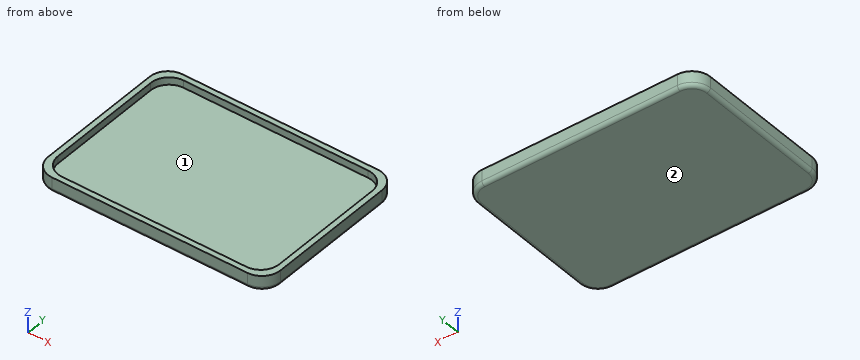
from build123d import *

# Parameters (mm, degrees)
F0_W     = 60
F0_H     = 42
F1_DEPTH = 2
F2_W     = 63
F2_H     = 45
F2_W_2   = 60
F2_H_2   = 42
F3_DEPTH = 4
F4_R     = 5
F5_R     = 1


with BuildPart() as f1:
    # F0 (on Top) → F1 (new body)
    with BuildSketch(Plane.XY):
        with Locations((30, 21)):
            Rectangle(F0_W, F0_H)
    extrude(amount=F1_DEPTH)

    # F2 (on Top) → F3 (join)
    with BuildSketch(Plane.XY):
        with Locations((30, 21)):
            Rectangle(F2_W, F2_H)
        with Locations((30, 21)):
            Rectangle(F2_W_2, F2_H_2, mode=Mode.SUBTRACT)
    extrude(amount=F3_DEPTH)

    # F4
    f4_edges = [f1.edges().sort_by_distance(p)[0] for p in [
        (-1.5, -1.5, 2),
        (61.5, -1.5, 2),
        (-1.5, 43.5, 2),
        (60, 42, 3),
        (61.5, 43.5, 2),
        (60, 0, 3),
        (0, 0, 3),
        (0, 42, 3),
    ]]
    fillet(f4_edges, radius=F4_R)

    # F5
    f5_edges = [f1.edges().sort_by_distance(p)[0] for p in [
        (30, -1.5, 0),
        (60.035534, -0.035534, 0),
        (61.5, 21, 0),
        (60.035534, 42.035534, 0),
        (30, 43.5, 0),
        (-0.035534, 42.035534, 0),
        (-1.5, 21, 0),
        (-0.035534, -0.035534, 0),
    ]]
    fillet(f5_edges, radius=F5_R)


solid = f1.part
Input: part model. Units: mm. Frame: model coordinates. Face numbers are marked on the shaded views. Round coordinates to 2 decimals unless told otherwise and drop trailing zeros. Order: outer loops, then holes, each group sorted by start corner. A loop starts at its lowest first (then second) coordinate and runs counter-clockwise, first axis right, second up.
1. Mould query, pull axis Y, two halves, no side actions, for the marked faces 1 and 2. Classes: released by +Y, released by -Y, zero draft, split by the parting line, or undercut.
The answers:
face 1: undercut
face 2: zero draft
2. Cut plane B-B, the plane x = 40. Output: boundary loops of the cut face in (y, z).
The answers:
outline: (-1.5, 1) arc R1 ccw to (-0.5, 0) - (42.5, 0) arc R1 ccw to (43.5, 1) - (43.5, 4) - (42, 4) - (42, 2) - (0, 2) - (0, 4) - (-1.5, 4) - close
3. Pin query (flat end, axial travel): P1, Ø10, axis at x = 47.5, y = 15, coming from the +Z side. Return the tip coordinate at first contact, or that it passes through.
The answers:
P1: stops at z = 2
4. Material intervals for line 1 (X direction, y = 24, z = 3.85); line 2 (Z direction, x = 43, y = 35); line 3 (Y direction, x = 29, z = 2.15), sorted ascending.
The answers:
line 1: x = -1.5 to 0, 60 to 61.5
line 2: z = 0 to 2
line 3: y = -1.5 to 0, 42 to 43.5
5. Cut plane A-A, the plane y = 30. Output: boundary loops of the cut face in (x, z), then the cut area to 3 significant figures.
The answers:
outline: (-1.5, 1) arc R1 ccw to (-0.5, 0) - (60.5, 0) arc R1 ccw to (61.5, 1) - (61.5, 4) - (60, 4) - (60, 2) - (0, 2) - (0, 4) - (-1.5, 4) - close
area: 132 mm2
